Autodesk Inventor part; units mm, degrees
ref_plane "YZ Plane" through (0, 0, 0) normal (1, 0, 0) x (0, 1, 0)
ref_plane "XZ Plane" through (0, 0, 0) normal (0, 1, 0) x (-1, 0, 0)
ref_plane "XY Plane" through (0, 0, 0) normal (0, 0, 1) x (1, 0, 0)
sketch "Sketch1" plane through (0, 0, 0) normal (0, 0, 1) x (1, 0, 0)
  line L0 (195, 300) -> (18, 300)
  line L1 (78, -2.5) -> (78, -18)
  line L2 (156, -2.5) -> (156, -18)
  line L3 (78, -18) -> (156, -18)
  line L4 (158.5, 0) -> (195, 0)
  line L5 (0, 0) -> (0, 75)
  line L6 (0, 150) -> (0, 225)
  line L7 (18, 300) -> (18, 227.5)
  line L8 (18, 147.5) -> (18, 77.5)
  line L9 (0, 0) -> (75.5, 0)
  arc A0 (15.5, 225) -> (18, 227.5) centre (18, 225) ccw
  line L10 (0, 225) -> (15.5, 225)
  arc A1 (18, 147.5) -> (15.5, 150) centre (18, 150) ccw
  line L11 (0, 150) -> (15.5, 150)
  arc A2 (15.5, 75) -> (18, 77.5) centre (18, 75) ccw
  line L12 (0, 75) -> (15.5, 75)
  arc A3 (78, -2.5) -> (75.5, 0) centre (78, 0) ccw
  arc A4 (158.5, 0) -> (156, -2.5) centre (156, 0) ccw
  line L13 (390, 150) -> (374.5, 150)
  arc A5 (374.5, 150) -> (372, 147.5) centre (372, 150) ccw
  line L14 (390, 225) -> (374.5, 225)
  line L15 (390, 150) -> (390, 225)
  arc A6 (372, 227.5) -> (374.5, 225) centre (372, 225) ccw
  line L16 (372, 147.5) -> (372, 77.5)
  line L17 (372, 300) -> (372, 227.5)
  line L18 (312, -2.5) -> (312, -18)
  line L19 (234, -2.5) -> (234, -18)
  line L20 (312, -18) -> (234, -18)
  line L21 (390, 75) -> (374.5, 75)
  line L22 (390, 0) -> (390, 75)
  line L23 (390, 0) -> (314.5, 0)
  arc A7 (314.5, 0) -> (312, -2.5) centre (312, 0) ccw
  arc A8 (234, -2.5) -> (231.5, 0) centre (234, 0) ccw
  arc A9 (372, 77.5) -> (374.5, 75) centre (372, 75) ccw
  line L24 (195, 300) -> (372, 300)
  line L25 (231.5, 0) -> (195, 0)
  dimension "d0" = 78
  dimension "d1" = 78
  dimension "d2" = 300
  dimension "d3" = 5
  dimension "d4" = 18
  dimension "d5" = 5
  dimension "d6" = 15.5
  dimension "d7" = 5
  dimension "d8" = 18
  dimension "d9" = 15.5
  dimension "d10" = 5
  dimension "d11" = 5
  dimension "d12" = 18
  dimension "d13" = 18
  dimension "d14" = 78
  dimension "d15" = 75
  dimension "d16" = 75
  dimension "d17" = 75
extrude "Extrusion1" add sketch "Sketch1" along normal blind 18
properties part number "cajon lat grande"
For this review, take the finished solid that the model builds, in its own axes (mm). A direction names the side the tool comes from. Coordinates: 2 decimals unless noted, no trailing zeros. Order: outer loops, then holes, each group sorted by start corner. A loop starts at its lowest first (then second) coordinate and runs counter-clockwise, first axis right, second up. Notation, with made-up numbers: (38, -27.75) - (93, -27.75) arc R14 ccw to (93, -15.75) - close; hole circle Ø11 at (-26, -37.5). An arc over 180 degrees is marked (long way). Answer as CSV lines item,"result". Start each with the question number.
1) Insertion check: P1, Ø5.5, axis at y = 269.5, z = 5.5, coming from the -X side; P2, Ø3, axis at x = 18, y = 225, coming from the -Z side; P3, Ø5, axis at x = 318.5, z = 12.5, coming from the -Y side; P4, Ø4.5, axis at x = 6.5, z = 13, coming from the +Y side. Each pin has a flat end and moves straight along its axis. Give the tip position at first contact, or say it passes through.
2) Draft analysis for pull direction X (two halves, no side actions). For faces 4 (the flat face through (234, -10, 9)), 5 (the flat face through (18, 264, 9)), 6 (the flat face through (382, 150, 9)), state which applies: +X half, -X half, draft (parallel to the pull), parting line (faces both ways), or undercut.
3) To check wall thickness, follow line 1 along Y through (x, z) = (188, 12); line 2 along X through (y, z) = (100.5, 6.5). State the ranges of each line that lie inside material, in increasing order. Write a range as [from, to].
4) Add section B-B (y = 134.5). State the section outline as (x, z) points.
5) Add section C-C (x = 180). State the section outline as (y, z) points, then the cut area to 3 significant figures.
6) Machinability: for faces 1 (the flat face through (8, 75, 9)), 2 (the flat face through (353, 0, 9)), 3 (the flat face through (196, 0, 9)), which of the approach directions +Z, -Z, +X, -X, +Y, -Y give a long, thin tool a straight path to every point of the face, cutting with its end or side? Answer none if there is none.
Result:
1,P1,"x = 18"
1,P2,"through"
1,P3,"y = 0"
1,P4,"y = 225"
2,face 4,"undercut"
2,face 5,"-X half"
2,face 6,"draft"
3,line 1,"[0, 300]"
3,line 2,"[18, 372]"
4,outline,"(18, 0) - (372, 0) - (372, 18) - (18, 18) - close"
5,outline,"(0, 0) - (300, 0) - (300, 18) - (0, 18) - close"
5,area,"5,400 mm^2"
6,face 1,"+Z, -Z, -X"
6,face 2,"+Z, -Z, +X, -Y"
6,face 3,"+Z, -Z, -Y"
